Here's how the part is built. I have some questions about the finished solid (model axes, mm). Face numbers are marked on the shaded views. A direction names the side the tool comes from. Give positions to 0.01 mm unless a question says otherwise; leave off trailing zeros. Loops run counter-clockwise (first coordinate to the right, second up) from the corner with the lowest first, then second, coordinate; pieces in that order, holes last. Notation, with made-up numbers: (75.25, 36.5) - (128.25, 36.5) arc R10 cw to (128.25, 42.5) - close; hole circle Ø11 at (37, -15.75). An arc over 180 degrees is marked (long way). Return JSON: item names as keys, results as strings. Group by question number.
(1) For P1, Ø2.5, axis at x = 0, y = 33.5, coming from the +Z side; P2, Ø1.2, axis at y = 27.5, z = 4, coming from the -X side; P3, Ø3, axis at x = 1, y = 15, coming from the -Z side, each with a flat end and sliding along its axis, tell me the tip position at first contact or that it passes through.
(2) If we section it at B-B (x = -33.5): Please give me the cut outline in (y, z).
(3) On a 3-axis mill with a long thin cutter (end or side, diameter ignored), from which of +Z, -Z, +X, -X, +Y, -Y can I reach the whole of each face in a straight line? I mean the marked faces 1 and 2. Say none if no direction works.
(4) If we section it at C-C (y = 25): Please give me the cut outline in (x, z), then the cut area to 3 significant figures.
(5) I need wall thicknesses on probe 1 along Y at (x, z) = (0, 3.2); probe 2 along X at (y, z) = (0, 0.9); probe 3 along Z at (x, y) = (-19.5, 6.5). Which ranges of each line are inside material? Lowest first, please. Write a range as [from, to].
(6) If we section it at A-A (z = 4.5): Please give me the cut outline in (x, y), then the cut area to 3 significant figures.
```python
from build123d import *

# Parameters (mm, degrees)
PAD_DEPTH       = 6
SKETCH001_W     = 28
SKETCH001_H     = 7.4
SKETCH001_W_2   = 7.4
SKETCH001_H_2   = 28
PAD001_DEPTH    = 0.4
SKETCH002_R     = 1.6
POCKET_DEPTH    = 6.401
SKETCH003_R     = 3
POCKET001_DEPTH = 1
PAD002_DEPTH    = 0.2
SKETCH007_R     = 1
POCKET002_DEPTH = 0.01
FILLET_R        = 2
CHAMFER_SIZE    = 0.4


with BuildPart() as part:
    # Sketch → Pad (new body)
    with BuildSketch(Plane.XY):
        with BuildLine():
            Line((-9.5, 40.5), (9.5, 40.5))
            Line((9.5, 40.5), (9.5, -9.5))
            Line((9.5, -9.5), (-40.5, -9.5))
            Line((-40.5, -9.5), (-40.5, 9.5))
            Line((-40.5, 9.5), (-18.5, 9.5))
            ThreePointArc((-18.5, 9.5), (-12.136039, 12.136039), (-9.5, 18.5))
            Line((-9.5, 18.5), (-9.5, 40.5))
        make_face()
    extrude(amount=PAD_DEPTH)

    # Sketch001 → Pad001 (new body)
    with BuildSketch(Plane.XY.offset(6)):
        with Locations((-25.5, 0)):
            Rectangle(SKETCH001_W, SKETCH001_H)
        with Locations((0, 25.5)):
            Rectangle(SKETCH001_W_2, SKETCH001_H_2)
    extrude(amount=PAD001_DEPTH)

    # Sketch002 → Pocket (cut, through all)
    with BuildSketch(Plane(origin=(0, 0, 0), x_dir=(1, 0, 0), z_dir=(0, 0, -1))):
        with Locations((-33.5, 0)):
            Circle(SKETCH002_R)
        with Locations((-16.5, 0)):
            Circle(SKETCH002_R)
        with Locations((0, -16.5)):
            Circle(SKETCH002_R)
        with Locations((0, -33.5)):
            Circle(SKETCH002_R)
        Circle(SKETCH002_R)
    extrude(amount=-POCKET_DEPTH, mode=Mode.SUBTRACT)

    # Sketch003 → Pocket001 (cut)
    with BuildSketch(Plane(origin=(0, 0, 0), x_dir=(1, 0, 0), z_dir=(0, 0, -1))):
        with Locations((-33.5, 0)):
            Circle(SKETCH003_R)
        with Locations((-16.5, 0)):
            Circle(SKETCH003_R)
        with Locations((0, -16.5)):
            Circle(SKETCH003_R)
        with Locations((0, -33.5)):
            Circle(SKETCH003_R)
        Circle(SKETCH003_R)
    extrude(amount=-POCKET001_DEPTH, mode=Mode.SUBTRACT)

    # Sketch006 → Pad002 (new body)
    with BuildSketch(Plane(origin=(0, 0, 1), x_dir=(1, 0, 0), z_dir=(0, 0, -1))):
        Polygon((-36.591786, 5.291606), (5.977032, 5.291606), (5.977032, -37.277212), (-5.613096, -37.277212), (-5.613096, -6.298522), (-36.591786, -6.298522), align=None)
    extrude(amount=-PAD002_DEPTH)

    # Sketch007 → Pocket002 (cut)
    with BuildSketch(Plane.XY.offset(6)):
        Circle(SKETCH007_R)
    extrude(amount=POCKET002_DEPTH, mode=Mode.SUBTRACT)

    # Fillet
    fillet_edges = [part.edges().sort_by_distance(p)[0] for p in [
        (-40.5, 9.5, 3),
        (-29.5, 9.5, 0),
        (-12.136039, 12.136039, 0),
        (-9.5, 29.5, 0),
        (0, 40.5, 0),
        (9.5, 15.5, 0),
        (9.5, -9.5, 3),
        (9.5, 40.5, 3),
        (-9.5, 40.5, 3),
        (-40.5, 0, 0),
        (-40.5, -9.5, 3),
        (-15.5, -9.5, 0),
    ]]
    fillet(fillet_edges, radius=FILLET_R)

    # Chamfer
    chamfer_edges = [part.edges().sort_by_distance(p)[0] for p in [
        (-19.5, 0, 0),
        (-36.5, 0, 0),
        (-3, 0, 0),
        (-3, 16.5, 0),
        (-3, 33.5, 0),
    ]]
    chamfer(chamfer_edges, length=CHAMFER_SIZE)


solid = part.part
```
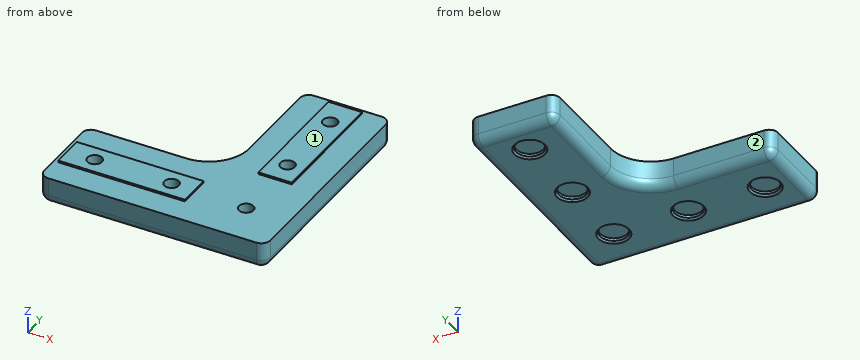
Values:
{
 "1": {"P1": "z = 1.2", "P2": "x = -9.5", "P3": "z = 0.1"},
 "2": {"outline": "(-9.5, 2) arc R2 ccw to (-7.5, 0) - (-3.4, 0) - (-3, 0.4) - (-3, 1) - (3, 1) - (3, 0.4) - (3.4, 0) - (7.5, 0) arc R2 ccw to (9.5, 2) - (9.5, 6) - (3.7, 6) - (3.7, 6.4) - (1.6, 6.4) - (1.6, 1.2) - (-1.6, 1.2) - (-1.6, 6.4) - (-3.7, 6.4) - (-3.7, 6) - (-9.5, 6) - close"},
 "3": {"face 1": "+Z, +X, -X, +Y, -Y", "face 2": "+Z, -Z, -X, +Y"},
 "4": {"outline": "(-9.5, 2) arc R2 ccw to (-7.5, 0) - (7.5, 0) arc R2 ccw to (9.5, 2) - (9.5, 6) - (3.7, 6) - (3.7, 6.4) - (-3.7, 6.4) - (-3.7, 6) - (-9.5, 6) - close", "area": "115 mm2"},
 "5": {"probe 1": "[-9.5, -1.6], [1.6, 14.9], [18.1, 31.9], [35.1, 40.5]", "probe 2": "[-40.17, -36.5], [-30.5, -19.5], [-13.5, -3], [3, 9.17]", "probe 3": "[0, 6]"},
 "6": {"outline": "(-40.5, -7.5) arc R2 ccw to (-38.5, -9.5) - (7.5, -9.5) arc R2 ccw to (9.5, -7.5) - (9.5, 38.5) arc R2 ccw to (7.5, 40.5) - (-7.5, 40.5) arc R2 ccw to (-9.5, 38.5) - (-9.5, 18.5) arc R9 cw to (-18.5, 9.5) - (-38.5, 9.5) arc R2 ccw to (-40.5, 7.5) - close; hole circle Ø3.2 at (-33.5, 0); hole circle Ø3.2 at (-16.5, 0); hole circle Ø3.2 at (0, 0); hole circle Ø3.2 at (0, 16.5); hole circle Ø3.2 at (0, 33.5)", "area": "1,510 mm2"}
}
